Input: part model. Units: mm. Frame: model coordinates. A direction names the side the tool comes from. Give positions to 0.01 mm unless a question says otherwise; leave off trailing zeros. Order: outer loops, then holes, each group sorted by start corner. A loop starts at its lowest first (then second) coordinate and runs counter-clockwise, first axis right, second up. Notation, with made-up numbers: (13.5, 47.25) - (22.5, 47.25) arc R20 cw to (22.5, 57.25) - close; hole circle Ø2 at (69, -27). An arc over 180 degrees is marked (long way). Answer in a Markdown table with one row per item. Add a question column.
1. Section query D-D on x = -26. Return loops of the section in (y, z).
2. Section query A-A on y = -45. Return loops of the section in (x, z).
3. Contact query for flat-ended pins moving along their axis: pin 1 (5.5 mm diameter, centred on y = -45, z = 0, fed in from -X); pin 2 (5 mm diameter, centred on x = -48.5, z = 25.5, fed in from -Y). Output: stop coordinate, or through.
4. Ray query, line 1 (X direction, y = -7.5, z = -2); line 2 (X direction, y = -8, z = -28); line 3 (Z direction, x = -59, y = -45). Return the intervals inside material, ascending. Write a range as [from, to].
5. Access query for faces 1 (the face through (57, -60, 0)), 2 (the face through (-52.5, -30, -21)), 3 (the face through (-54.965, -18.89, -6.944)). Directions: +Z, -Z, +X, -X, +Y, -Y. A direction counts if a zero-diameter tool reaches every point of the face in a straight line with its end or side. Return the directions, or none.
6. Section query B-B on y = -37.5. Return loops of the section in (x, z), and give its area (3 significant figures).
7. Mould query, pull axis X, two halves, no side actions, for faces 4 (the face through (52.5, -30, 0)), 5 (the face through (0, 1, -35)). Classes: released by +X, released by -X, zero draft, split by the parting line, or undercut.
8. Section query C-C on z = -27.5. Return loops of the section in (x, y).
```python
from build123d import *

# Parameters (mm, degrees)
SKETCH2_W           = 125
SKETCH2_H           = 70
BOSS_EXTRUDE1_DEPTH = 10
SKETCH3_W           = 10
SKETCH3_H           = 70
BOSS_EXTRUDE2_DEPTH = 60
CUT_EXTRUDE1_DEPTH  = 5
CUT_EXTRUDE2_START  = -15
SKETCH6_R           = 3.5
CUT_EXTRUDE2_DEPTH  = 15


with BuildPart() as part:
    # Sketch2 → Boss-Extrude1 (new body)
    with BuildSketch(Plane(origin=(0, 0, 0), x_dir=(1, 0, 0), z_dir=(0, 1, 0))):
        Rectangle(SKETCH2_W, SKETCH2_H)
    extrude(amount=BOSS_EXTRUDE1_DEPTH)

    # Sketch3 → Boss-Extrude2 (add)
    with BuildSketch(Plane.XZ):
        with Locations((-57.5, 0)):
            Rectangle(SKETCH3_W, SKETCH3_H)
        with Locations((57.5, 0)):
            Rectangle(SKETCH3_W, SKETCH3_H)
    extrude(amount=BOSS_EXTRUDE2_DEPTH)

    # Sketch4 → Cut-Extrude1 (cut)
    with BuildSketch(Plane(origin=(-52.5, 0, 0), x_dir=(0, 0, -1), z_dir=(1, 0, 0))):
        with BuildLine():
            Line((-3.395932152, -60), (-0.813446687, -60))
            Line((-0.813446687, -60), (1.422755234, -48.197775406))
            ThreePointArc((1.422755234, -48.197775406), (-3.43881752, -44.348437214), (2.493929957, -42.544330362))
            Line((2.493929957, -42.544330362), (4.2626708, -33.209271445))
            ThreePointArc((4.2626708, -33.209271445), (6.134370688, -31.923293743), (7.636341499, -30.220037214))
            Line((7.636341499, -30.220037214), (23.57750665, -29.157373753))
            ThreePointArc((23.57750665, -29.157373753), (26.139587656, -26.579311787), (23.90653542, -23.711535594))
            Line((23.90653542, -23.711535594), (8.209271445, -20.7373292))
            ThreePointArc((8.209271445, -20.7373292), (6.923293743, -18.865629312), (5.220037214, -17.363658501))
            Line((5.220037214, -17.363658501), (4.062548081, 0))
            Line((4.062548081, 0), (-1.081282483, 0))
            Line((-1.081282483, 0), (-4.2626708, -16.790728555))
            ThreePointArc((-4.2626708, -16.790728555), (-6.134370688, -18.076706257), (-7.636341499, -19.779962786))
            Line((-7.636341499, -19.779962786), (-23.57750665, -20.842626247))
            ThreePointArc((-23.57750665, -20.842626247), (-26.139587656, -23.420688213), (-23.90653542, -26.288464406))
            Line((-23.90653542, -26.288464406), (-8.209271445, -29.2626708))
            ThreePointArc((-8.209271445, -29.2626708), (-6.923293743, -31.134370688), (-5.220037214, -32.636341499))
            Line((-5.220037214, -32.636341499), (-3.395932152, -60))
        make_face()
    extrude(amount=-CUT_EXTRUDE1_DEPTH, mode=Mode.SUBTRACT)

    # Sketch6 → Cut-Extrude2 (cut)
    with BuildSketch(Plane.ZY.offset(62.5).offset(CUT_EXTRUDE2_START)):
        with Locations((0, -45)):
            Circle(SKETCH6_R)
    extrude(amount=CUT_EXTRUDE2_DEPTH, mode=Mode.SUBTRACT)


solid = part.part
```
Answer:
| question | item | result |
|---|---|---|
| 1 | outline | (0, -35) - (10, -35) - (10, 35) - (0, 35) - close |
| 2 | outline | (-62.5, -35) - (-52.5, -35) - (-52.5, -3.5) - (-62.5, -3.5) - close; (-62.5, 3.5) - (-57.5, 3.5) - (-57.5, 4.4) - (-52.5, 4.4) - (-52.5, 35) - (-62.5, 35) - close; (52.5, -35) - (62.5, -35) - (62.5, 35) - (52.5, 35) - close |
| 3 | pin 1 | stops at x = 52.5 |
| 3 | pin 2 | stops at y = 0 |
| 4 | line 1 | x = [-62.5, -57.5], [52.5, 62.5] |
| 4 | line 2 | x = [-62.5, -52.5], [52.5, 62.5] |
| 4 | line 3 | z = [-35, -3.5], [3.5, 35] |
| 5 | face 1 | +Z, -Z, +X, -X, -Y |
| 5 | face 2 | +Z, -Z, -Y |
| 5 | face 3 | none |
| 6 | outline | (-62.5, -35) - (-52.5, -35) - (-52.5, -3.45) - (-57.5, -3.45) - (-57.5, 4.9) - (-52.5, 4.9) - (-52.5, 35) - (-62.5, 35) - close; (52.5, -35) - (62.5, -35) - (62.5, 35) - (52.5, 35) - close |
| 6 | area | 1,360 mm² |
| 7 | face 4 | undercut |
| 7 | face 5 | zero draft |
| 8 | outline | (-62.5, -60) - (-52.5, -60) - (-52.5, 0) - (52.5, 0) - (52.5, -60) - (62.5, -60) - (62.5, 10) - (-62.5, 10) - close |
